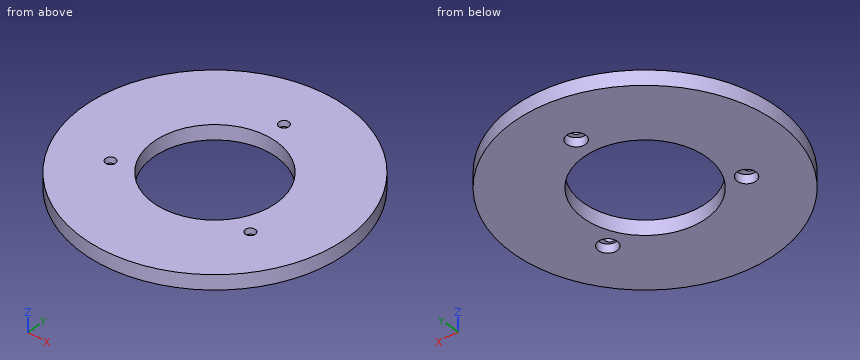
from build123d import *

# Parameters (mm, degrees)
CROQUIS1_R                   = 45
CROQUIS1_R_2                 = 21
SALIENTE_EXTRUIR1_DEPTH      = 5
TALADRO_DE_MARGEN_PARA_M31_D = 3.4
CROQUIS4_R                   = 3.2
CORTAR_EXTRUIR1_DEPTH        = 3


with BuildPart() as part:
    # Croquis1 → Saliente-Extruir1 (new body)
    with BuildSketch(Plane.XY):
        Circle(CROQUIS1_R)
        Circle(CROQUIS1_R_2, mode=Mode.SUBTRACT)
    extrude(amount=SALIENTE_EXTRUIR1_DEPTH)

    # Taladro de margen para M31 (through all)
    with Locations(Plane(origin=(0, 0, 0), x_dir=(-1, 0, 0), z_dir=(0, 0, -1))):
        with Locations((0, 27.75), (24.032204955, -13.875), (-24.032204955, -13.875)):
            Hole(TALADRO_DE_MARGEN_PARA_M31_D / 2)

    # Croquis4 → Cortar-Extruir1 (cut)
    with BuildSketch(Plane(origin=(0, 0, 0), x_dir=(-1, 0, 0), z_dir=(0, 0, -1))):
        with Locations((0, 27.75)):
            Circle(CROQUIS4_R)
        with Locations((23.382685902, -13.5)):
            Circle(CROQUIS4_R)
        with Locations((-24.032204955, -13.125)):
            Circle(CROQUIS4_R)
    extrude(amount=-CORTAR_EXTRUIR1_DEPTH, mode=Mode.SUBTRACT)


solid = part.part
Check sheet for the modelled part. Datum: model origin and axes. Units: mm. Round coordinates to 2 decimals unless told otherwise and drop trailing zeros. Write each loop counter-clockwise with the first axis right and the second up, starting at its lowest first coordinate (ties: lowest second). Pieces come first, ordered by that corner, then holes. Notation, with made-up numbers: (-10.5, -30) - (25.5, -30) arc R10 cw to (25.5, -18) - close; hole circle Ø2 at (72.5, 71). An arc over 180 degrees is marked (long way). Return JSON: item names as keys, results as strings.
Q1. Cross-section at C-C (z = 1.2). Record the boundary of the cut face in (x, y) (3 decimals).
Returned:
{"outline": "circle Ø90 at (0, 0); hole circle Ø6.4 at (-23.383, -13.5); hole circle Ø42 at (0, 0); hole circle Ø6.4 at (0, 27.75); hole circle Ø6.4 at (24.032, -13.125)"}
Q2. Scan lines: L1, parallel to Y at x = 0, z = 1.8; L2, parallel to Y at x = 0, z = 4.4; L3, parallel to Y at x = -11, z = 2.7. Record each from-to range of solid material in increasing order. Write a range as from..to.
Returned:
{"L1": "y = -45..-21, 21..24.55, 30.95..45", "L2": "y = -45..-21, 21..26.05, 29.45..45", "L3": "y = -43.63..-17.89, 17.89..43.63"}
Q3. Cross-section at D-D (x = -24). Record the boundary of the cut face in (y, z), then the cut area to 3 significant figures.
Returned:
{"outline": "(-38.07, 0) - (-16.64, 0) - (-16.64, 3) - (-15.57, 3) - (-15.57, 5) - (-38.07, 5) - close; (-12.18, 3) - (-10.36, 3) - (-10.36, 0) - (38.07, 0) - (38.07, 5) - (-12.18, 5) - close", "area": "355 mm²"}
Q4. Cross-section at A-A (y = 0). Record the boundary of the cut face in (x, z), then the cut area to 3 significant figures.
Returned:
{"outline": "(-45, 0) - (-21, 0) - (-21, 5) - (-45, 5) - close; (21, 0) - (45, 0) - (45, 5) - (21, 5) - close", "area": "240 mm²"}
Q5. Depth check by flat-ended pin: P1, Ø1, axis at y = -6.5, z = 4, coming from the +X side; P2, Ø6, axis at x = -23.38, y = -13.5, coming from the -Z side; P3, Ø2, axis at x = 14, z = 2, coming from the -Y side. Enter the tip coordinate at first touch or a pass-through.
Returned:
{"P1": "stops at x = 44.6", "P2": "stops at z = 3", "P3": "stops at y = -43.08"}
Q6. Cross-section at B-B (x = 0). Record the boundary of the cut face in (y, z), then the cut area to 3 significant figures.
Returned:
{"outline": "(-45, 0) - (-21, 0) - (-21, 5) - (-45, 5) - close; (21, 0) - (24.55, 0) - (24.55, 3) - (26.05, 3) - (26.05, 5) - (21, 5) - close; (29.45, 3) - (30.95, 3) - (30.95, 0) - (45, 0) - (45, 5) - (29.45, 5) - close", "area": "214 mm²"}
